Can you work these out from the model? Positions are in its coordinate system, mm. Face numbers are marked on the shaded views. A direction names the side the tool comes from. Give positions to 0.01 mm unless a question says otherwise; leave off trailing zeros. Loops run counter-clockwise (first coordinate to the right, second up) from the corner with the lowest first, then second, coordinate; pieces in that order, holes last. Notation, with made-up numbers: M 27,76 L 50,76 A13 ccw 50,92 Z; hole C 74.25,20.25 d2. An arc over 180 degrees is marked long. Put each result on its own line as item: value. Start each with the question number.
1) Imagine slicing it at D-D (z = 1.25). Write out the boundary of the cut face in (x, y).
2) For P1, Ø3, axis at x = 1, y = 0, coming from the +Z side; P2, Ø1.5, axis at x = -4, z = 3, coming from the +Y side; P3, Ø3, axis at x = -1.5, y = -1.5, coming from the +Z side, each with a flat end and sliding along its axis, tell me the tip position at first contact or that it passes through.
3) Imagine slicing it at C-C (z = 2.75). Write out the boundary of the cut face in (x, y).
4) Please list where these lines run through material, in increasing order: line 1 along Y through (x, z) = (0, 0.6); line 2 along Y through (x, z) = (0, 3.25); line 3 along X through (y, z) = (2.5, 2.25). Write a range as from..to.
5) If we mould it in two halves opening along Y, with no side actions, what happens to the marked faces 1, 2 and 3? For each: +Y half, -Y half, draft (parallel to the pull), parting line (faces both ways), or undercut.
6) For the marked faces 4 and 5, which set-ups out of +Z, -Z, +X, -X, +Y, -Y let a thin tool reach every point of the face, with its end or its side?
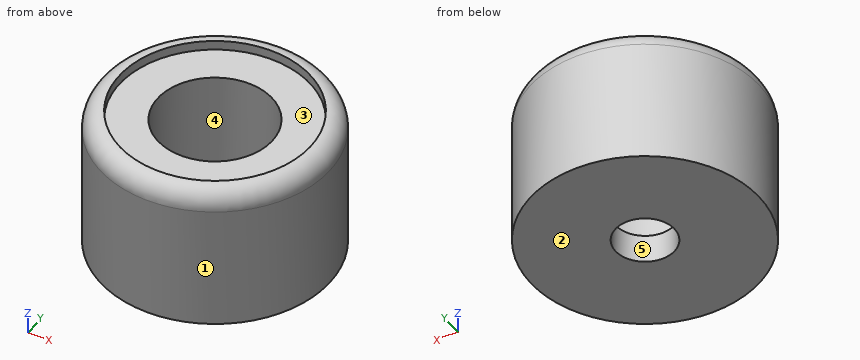
from build123d import *

# Parameters (mm, degrees)
SKETCH1_R           = 3
SKETCH1_R_2         = 1.55
BOSS_EXTRUDE1_DEPTH = 1.5
SKETCH1_7_R         = 5
SKETCH1_7_R_2       = 3
BOSS_EXTRUDE3_DEPTH = 7
SKETCH1_9_R         = 6
SKETCH1_9_R_2       = 5
BOSS_EXTRUDE4_DEPTH = 7.5
FILLET1_R           = 1


with BuildPart() as part:
    # Sketch1 → Boss-Extrude1 (new body)
    with BuildSketch(Plane.XY):
        Circle(SKETCH1_R)
        Circle(SKETCH1_R_2, mode=Mode.SUBTRACT)
    extrude(amount=BOSS_EXTRUDE1_DEPTH)

    # Sketch1<7> → Boss-Extrude3 (add)
    with BuildSketch(Plane.XY):
        Circle(SKETCH1_7_R)
        Circle(SKETCH1_7_R_2, mode=Mode.SUBTRACT)
    extrude(amount=BOSS_EXTRUDE3_DEPTH)

    # Sketch1<9> → Boss-Extrude4 (add)
    with BuildSketch(Plane.XY):
        Circle(SKETCH1_9_R)
        Circle(SKETCH1_9_R_2, mode=Mode.SUBTRACT)
    extrude(amount=BOSS_EXTRUDE4_DEPTH)

    # Fillet1
    fillet1_edges = [part.edges().sort_by_distance(p)[0] for p in [
        (-6, 0, 7.5),
    ]]
    fillet(fillet1_edges, radius=FILLET1_R - 0.0001)  # a hair under: the kernel refuses the full size


solid = part.part
Recorded:
1. outline: C 0,0 d12; hole C 0,0 d3.1
2. P1: z = 1.5
2. P2: y = 5.04
2. P3: z = 7
3. outline: C 0,0 d12; hole C 0,0 d6
4. line 1: -6..-1.55, 1.55..6
4. line 2: -6..-3, 3..6
4. line 3: -5.45..-1.66, 1.66..5.45
5. face 1: parting line
5. face 2: draft
5. face 3: undercut
6. face 4: +Z
6. face 5: +Z, -Z
